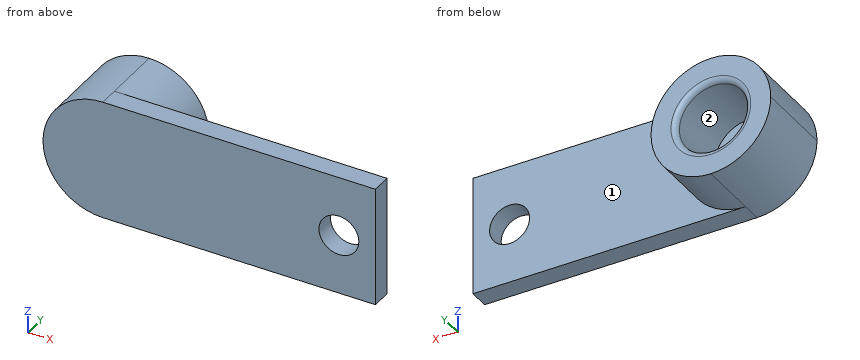
```python
from build123d import *

# Parameters (mm, degrees)
SKETCH2_W               = 25
SKETCH2_H               = 9
BOSS_EXTRUDE3_DEPTH     = 6
SKETCH3_R               = 2.6
CUT_EXTRUDE1_DEPTH      = 5
CUT_EXTRUDE2_DEPTH      = 28.239676944
CUT_EXTRUDE2_DEPTH_BACK = 28.239676944
SKETCH4_R               = 1.5
SKETCH5_R               = 1.5
CUT_EXTRUDE3_DEPTH      = 4.5
CUT_EXTRUDE4_DEPTH      = 28.239676944
FILLET2_R               = 0.4


with BuildPart() as part:
    # Sketch2 → Boss-Extrude3 (new body)
    with BuildSketch(Plane(origin=(0, 0, 0), x_dir=(1, 0, 0), z_dir=(0, 1, 0))):
        with Locations((12.5, 4.5)):
            Rectangle(SKETCH2_W, SKETCH2_H)
    extrude(amount=BOSS_EXTRUDE3_DEPTH)

    # Sketch3 → Cut-Extrude1 (cut)
    with BuildSketch(Plane(origin=(0, 6, 0), x_dir=(1, 0, 0), z_dir=(0, 1, 0))):
        with Locations(Location((4.5, 4.5, 0), (0, 0, 270))):
            Circle(SKETCH3_R)
    extrude(amount=-CUT_EXTRUDE1_DEPTH, mode=Mode.SUBTRACT)

    # Sketch4 → Cut-Extrude2 (cut, two sides: drawn at the far end of the back side and taken through both)
    with BuildSketch(Plane(origin=(0, 6, 0), x_dir=(1, 0, 0), z_dir=(0, 1, 0)).offset(-CUT_EXTRUDE2_DEPTH_BACK)):
        with Locations(Location((22.25, 4.5, 0), (0, 0, 270))):
            Circle(SKETCH4_R)
    extrude(amount=CUT_EXTRUDE2_DEPTH + CUT_EXTRUDE2_DEPTH_BACK, mode=Mode.SUBTRACT)

    # Sketch5 → Cut-Extrude3 (cut)
    with BuildSketch(Plane(origin=(0, 6, 0), x_dir=(1, 0, 0), z_dir=(0, 1, 0))):
        with BuildLine():
            Line((25, 9), (4.5, 9))
            ThreePointArc((4.5, 9), (7.681980515, 7.681980515), (9, 4.5))
            ThreePointArc((9, 4.5), (7.681980515, 1.318019485), (4.5, 0))
            Line((4.5, 0), (25, 0))
            Line((25, 0), (25, 9))
        make_face()
        with Locations(Location((22.25, 4.5, 0), (0, 0, 270))):
            Circle(SKETCH5_R, mode=Mode.SUBTRACT)
    extrude(amount=-CUT_EXTRUDE3_DEPTH, mode=Mode.SUBTRACT)

    # Sketch6 → Cut-Extrude4 (cut, through all)
    with BuildSketch(Plane(origin=(0, 6, 0), x_dir=(1, 0, 0), z_dir=(0, 1, 0))):
        with BuildLine():
            ThreePointArc((0, 4.5), (1.318019485, 7.681980515), (4.5, 9))
            Line((4.5, 9), (0, 9))
            Line((0, 9), (0, 4.5))
        make_face()
        with BuildLine():
            ThreePointArc((4.5, 0), (1.318019485, 1.318019485), (0, 4.5))
            Line((0, 4.5), (0, 0))
            Line((0, 0), (4.5, 0))
        make_face()
    extrude(amount=-CUT_EXTRUDE4_DEPTH, mode=Mode.SUBTRACT)

    # Fillet2
    fillet2_edges = [part.edges().sort_by_distance(p)[0] for p in [
        (4.5, 6, -7.1),
    ]]
    fillet(fillet2_edges, radius=FILLET2_R)


solid = part.part
```
Verification items for the finished model (mm, model axes). Face numbers are marked on the shaded views. Coordinates: 2 decimals unless noted, no trailing zeros. Order: outer loops, then holes, each group sorted by start corner. A loop starts at its lowest first (then second) coordinate and runs counter-clockwise, first axis right, second up. Notation, with made-up numbers: (41.5, -28.75) -> (63.5, -28.75) arc R25 cw to (63.5, -14.75) -> close; hole circle Ø7 at (27, 87.25). An arc over 180 degrees is marked (long way). Answer as CSV lines item,"result". Start each with the question number.
1) Material ranges on L1, parallel to Z at x = 22.25, y = 0.65; L2, parallel to X at y = 0.8, z = -4.5; L3, parallel to X at y = 2.8, z = -4.5, recorded low to high. Write a range as [from, to].
2) Cross-section at A-A, the plane x = 22.25. Record the boundary of the cut face in (y, z), then the cut area to 3 significant figures.
3) Release check for a two-part mould opening along Z. For the marked faces 1 and 2 record: released by +Z, released by -Z, zero draft, split by the parting line, or undercut.
4) Cross-section at B-B, the plane z = -8.25. Record the boundary of the cut face in (x, y).
5) Gauge pin test, flat ends, axial feed: pin 1 Ø1.5 at (x, z) = (3.5, -5.5) entering from +Y; pin 2 Ø4 at (x, z) = (20, -6.5) entering from +Y; pin 3 Ø3.5 at (x, z) = (22.25, -4.5) entering from -Y. Record the tip position at first contact, or that the pin passes through.
Conclusion:
1,L1,"z = [-9, -6], [-3, 0]"
1,L2,"x = [0, 20.75], [23.75, 25]"
1,L3,"x = [0, 1.9], [7.1, 9]"
2,outline,"(0, -9) -> (1.5, -9) -> (1.5, -6) -> (0, -6) -> close; (0, -3) -> (1.5, -3) -> (1.5, 0) -> (0, 0) -> close"
2,area,"9.00 mm²"
3,face 1,"zero draft"
3,face 2,"undercut"
4,outline,"(2.01, 0) -> (25, 0) -> (25, 1.5) -> (6.99, 1.5) -> (6.99, 6) -> (2.01, 6) -> close"
5,pin 1,"stops at y = 1"
5,pin 2,"stops at y = 1.5"
5,pin 3,"stops at y = 0"
